from build123d import *

# Parameters (mm, degrees)
SKETCH1_W                    = 72.898
SKETCH1_H                    = 19.05
SKETCH1_R                    = 4.191
BOSS_EXTRUDE1_DEPTH          = 1.27
SKETCH7_W                    = 72.898
SKETCH7_H                    = 1.27
BOSS_EXTRUDE4_DEPTH          = 30.48
CUT_EXTRUDE2_DEPTH           = 50.267816331
SKETCH10_W                   = 1.27
SKETCH10_H                   = 27.94
BOSS_EXTRUDE5_DEPTH          = 8.89
SKETCH11_W                   = 1.27
SKETCH11_H                   = 27.94
BOSS_EXTRUDE6_DEPTH          = 11.43
SKETCH12_R                   = 2.5
CUT_EXTRUDE3_DEPTH           = 72.631264997
CUT_EXTRUDE5_DEPTH           = 72.631264997
CUT_EXTRUDE5_DEPTH_BACK      = 72.631264997
SKETCH14_W                   = 12.7
SKETCH14_H                   = 5.24
SKETCH15_W                   = 36.322
SKETCH15_H                   = 1.27
BOSS_EXTRUDE8_DEPTH          = 3.81
BOSS_EXTRUDE9_START          = 29.05
BOSS_EXTRUDE9_DEPTH          = 1.27
SKETCH17_R                   = 4.191
CUT_EXTRUDE6_DEPTH           = 1.27
CUT_EXTRUDE6_DRAFT           = -60
CUT_EXTRUDE6_PROFILE_2_DEPTH = 1.27
CUT_EXTRUDE6_PROFILE_2_DRAFT = -60


with BuildPart() as part:
    # Sketch1 → Boss-Extrude1 (new body)
    # profile 1 of 3: a face of its own
    with BuildSketch(Plane(origin=(0, 0, 0), x_dir=(1, 0, 0), z_dir=(0, 1, 0))):
        Rectangle(SKETCH1_W, SKETCH1_H)
        with Locations((28.829, 1.905)):
            Circle(SKETCH1_R, mode=Mode.SUBTRACT)
        with Locations((-28.829, 1.905)):
            Circle(SKETCH1_R, mode=Mode.SUBTRACT)
    # profile 2 of 3: a face of its own
    with BuildSketch(Plane(origin=(0, 0, 0), x_dir=(1, 0, 0), z_dir=(0, 1, 0))):
        with Locations((28.829, 1.905)):
            Circle(SKETCH1_R)
    # profile 3 of 3: a face of its own
    with BuildSketch(Plane(origin=(0, 0, 0), x_dir=(1, 0, 0), z_dir=(0, 1, 0))):
        with Locations((-28.829, 1.905)):
            Circle(SKETCH1_R)
    extrude(amount=BOSS_EXTRUDE1_DEPTH)

    # Cut-Extrude1 cone 1 section (through the dimple's axis) → Cut-Extrude1 (revolve, cut)
    with BuildSketch(Plane(origin=(-28.829, 0, -1.905), x_dir=(0, 0, -1), z_dir=(1, 0, 0))):
        Polygon((0, 0), (4.191, 0), (0, 2.419674978), align=None)
    revolve(axis=Axis((-28.829, 0, -1.905), (0, 1, 0)), mode=Mode.SUBTRACT)

    # Cut-Extrude1 cone 2 section (through the dimple's axis) → Cut-Extrude1 cone 2 (revolve, cut)
    with BuildSketch(Plane(origin=(28.829, 0, -1.905), x_dir=(0, 0, -1), z_dir=(1, 0, 0))):
        Polygon((0, 0), (4.191, 0), (0, 2.419674978), align=None)
    revolve(axis=Axis((28.829, 0, -1.905), (0, 1, 0)), mode=Mode.SUBTRACT)

    # Sketch7 → Boss-Extrude4 (add)
    with BuildSketch(Plane(origin=(0, 1.27, 0), x_dir=(1, 0, 0), z_dir=(0, 1, 0))):
        with Locations((0, -8.89)):
            Rectangle(SKETCH7_W, SKETCH7_H)
    extrude(amount=BOSS_EXTRUDE4_DEPTH)

    # Sketch8 → Cut-Extrude2 (cut, symmetric)
    with BuildSketch(Plane.XZ):
        Polygon((-36.449, 9.525), (-36.449, 3.354745169), (-18.161, 8.255), (-18.161, 9.525), align=None)
    cut_extrude2 = extrude(amount=CUT_EXTRUDE2_DEPTH, both=True, mode=Mode.SUBTRACT)

    # Mirror2: Cut-Extrude2 across plane
    add(cut_extrude2.mirror(Plane.ZY), mode=Mode.SUBTRACT)

    # Sketch10 → Boss-Extrude5 (add)
    with BuildSketch(Plane.ZY.offset(18.161)):
        with Locations((8.89, 17.78)):
            Rectangle(SKETCH10_W, SKETCH10_H)
    extrude(amount=BOSS_EXTRUDE5_DEPTH)

    # Sketch11 → Boss-Extrude6 (add)
    with BuildSketch(Plane(origin=(0, 0, 8.255), x_dir=(-1, 0, 0), z_dir=(0, 0, -1))):
        with Locations((26.416, 17.78)):
            Rectangle(SKETCH11_W, SKETCH11_H)
    extrude(amount=BOSS_EXTRUDE6_DEPTH)

    # Sketch12 → Cut-Extrude3 (cut, through all)
    with BuildSketch(Plane.ZY.offset(27.051)):
        with Locations((2.77876, 10.16)):
            Circle(SKETCH12_R)
        with Locations((2.77876, 20.16)):
            Circle(SKETCH12_R)
    extrude(amount=-CUT_EXTRUDE3_DEPTH, mode=Mode.SUBTRACT)

    # Sketch14 → Cut-Extrude5 (cut, two sides: drawn at the far end of the back side and taken through both)
    with BuildSketch(Plane.ZY.offset(27.051).offset(-CUT_EXTRUDE5_DEPTH_BACK)):
        with Locations((3.175, 29.13)):
            Rectangle(SKETCH14_W, SKETCH14_H)
    extrude(amount=CUT_EXTRUDE5_DEPTH + CUT_EXTRUDE5_DEPTH_BACK, mode=Mode.SUBTRACT)

    # Sketch15 → Boss-Extrude8 (add)
    with BuildSketch(Plane(origin=(0, 26.51, 0), x_dir=(1, 0, 0), z_dir=(0, 1, 0))):
        with Locations((0, -8.89)):
            Rectangle(SKETCH15_W, SKETCH15_H)
    extrude(amount=BOSS_EXTRUDE8_DEPTH)

    # Sketch16 → Boss-Extrude9 (add)
    with BuildSketch(Plane(origin=(0, 1.27, 0), x_dir=(1, 0, 0), z_dir=(0, 1, 0)).offset(BOSS_EXTRUDE9_START)):
        Polygon((-36.449, 9.525), (-36.449, -3.354745169), (-18.161, -8.255), (-18.161, -9.525), (18.161, -9.525), (18.161, -8.255), (36.449, -3.354745169), (36.449, 9.525), align=None)
    extrude(amount=-BOSS_EXTRUDE9_DEPTH)


with BuildPart() as cut_extrude6_tool:
    # Sketch17 → Cut-Extrude6 (with draft: the straight prism first)
    with BuildSketch(Plane(origin=(0, 30.32, 0), x_dir=(1, 0, 0), z_dir=(0, 1, 0))):
        with Locations((-28.829, 1.905)):
            Circle(SKETCH17_R)
    extrude(amount=-CUT_EXTRUDE6_DEPTH)
    # Cut-Extrude6: the draft: its side faces are tilted about the plane it starts from
    cut_extrude6_sides = [cut_extrude6_tool.faces().sort_by_distance(p)[0] for p in [
        (-33.02, 29.685, -1.905),
    ]]
    draft(cut_extrude6_sides, Plane(origin=(0, 30.32, 0), x_dir=(1, 0, 0), z_dir=(0, 1, 0)), CUT_EXTRUDE6_DRAFT)


with BuildPart() as part_1:
    add(part.part)

    # Cut-Extrude6: cut by cut_extrude6_tool
    add(cut_extrude6_tool.part, mode=Mode.SUBTRACT)


with BuildPart() as cut_extrude6_profile_2_tool:
    # Sketch17 → Cut-Extrude6 profile 2 (with draft: the straight prism first)
    with BuildSketch(Plane(origin=(0, 30.32, 0), x_dir=(1, 0, 0), z_dir=(0, 1, 0))):
        with Locations((28.829, 1.905)):
            Circle(SKETCH17_R)
    extrude(amount=-CUT_EXTRUDE6_PROFILE_2_DEPTH)
    # Cut-Extrude6 profile 2: the draft: its side faces are tilted about the plane it starts from
    cut_extrude6_profile_2_sides = [cut_extrude6_profile_2_tool.faces().sort_by_distance(p)[0] for p in [
        (24.638, 29.685, -1.905),
    ]]
    draft(cut_extrude6_profile_2_sides, Plane(origin=(0, 30.32, 0), x_dir=(1, 0, 0), z_dir=(0, 1, 0)), CUT_EXTRUDE6_PROFILE_2_DRAFT)


with BuildPart() as part_2:
    add(part_1.part)

    # Cut-Extrude6 profile 2: cut by cut_extrude6_profile_2_tool
    add(cut_extrude6_profile_2_tool.part, mode=Mode.SUBTRACT)


solid = part_2.part
Verification items for the finished model (mm, model axes). A direction names the side the tool comes from. Give positions to 0.01 mm unless a question says otherwise; leave off trailing zeros. Loops run counter-clockwise (first coordinate to the right, second up) from the corner with the lowest first, then second, coordinate; pieces in that order, holes last. Notation, with made-up numbers: (-11, -38.75) - (16, -38.75) arc R6 ccw to (16, -33.75) - close; hole circle Ø5 at (83.5, -30.75). An arc over 180 degrees is marked (long way). Write item = value, one per line. Start each with the question number.
Q1. Cross-section at D-D, the plane y = 17. Enter the section's corners in (x, z) (3 decimals).
Q2. Cross-section at C-C, the plane x = -14. Enter the section's corners in (y, z) (3 decimals), and give its area (3 significant figures).
Q3. Mould release check, pull along Y, two halves, no side actions. Record for faces 6 (the face through (-26.425, 8.639, 0.795)), 7 (the face through (-1, 0, 0)), 8 (the face through (-36.449, 30, -3)): released by +Y, released by -Y, zero draft, split by the parting line, or undercut.
Q4. Cross-section at A-A, the plane z = -7.25. Enter the section's corners in (x, y), and give its area (3 significant figures).
Q5. Thickness scan on line 1 (Y direction, x = -20, z = -7); line 2 (Y direction, x = -26.5, z = 5.75); line 3 (X direction, y = 11.5, z = 6.75). Record the ranges inside material, lowest first.
Q6. Depth check by flat-ended pin: P1, Ø1.5, axis at x = -10, z = 5.5, coming from the -Y side; P2, Ø2, axis at x = -29, y = 8, coming from the -Z side; P3, Ø1.4, axis at y = 2.5, z = 9, coming from the -X side; P4, Ø5, axis at x = 20.5, y = 23, coming from the -Z side (3 decimals). Enter the tip coordinate at first touch or a pass-through.
Q7. Cross-section at B-B, the plane y = 10.16. Enter the section's corners in (x, z) (3 decimals).
Q8. Tool access check on faces 1 (the face through (-18.161, 28, 9)), 2 (the face through (-26.42, 22.64, 2.45)), 3 (the face through (-25.781, 15, 3)), 4 (the face through (-1, 1.27, -1)), 5 (the face through (-26, 26.51, 5)). Record the directions out of +Z, -Z, +X, -X, +Y, -Y that give a thin tool (end or side, any length) a straight path to the whole face; none if there is none.
Answer key:
q1.outline = (-27.051, -3.175) - (-25.781, -3.175) - (-25.781, 8.255) - (18.161, 8.255) - (18.161, 9.525) - (-27.051, 9.525) - close
q2.outline = (0, -9.525) - (1.27, -9.525) - (1.27, 8.255) - (29.05, 8.255) - (29.05, -9.525) - (30.32, -9.525) - (30.32, 9.525) - (0, 9.525) - close
q2.area = 83.7 mm^2
q3.face_6 = undercut
q3.face_7 = released by -Y
q3.face_8 = zero draft
q4.outline = (-36.45, 0) - (36.45, 0) - (36.45, 1.27) - (-36.45, 1.27) - close; (-36.45, 29.05) - (36.45, 29.05) - (36.45, 30.32) - (-36.45, 30.32) - close
q4.area = 185 mm^2
q5.line_1 = 0 to 1.27, 29.05 to 30.32
q5.line_2 = 0 to 1.27, 3.81 to 26.51, 29.05 to 30.32
q5.line_3 = -27.05 to -25.78
q6.P1 = 0
q6.P2 = through
q6.P3 = -18.16
q6.P4 = 8.255
q7.outline = (-27.051, -3.175) - (-25.781, -3.175) - (-25.781, 0.279) - (-27.051, 0.279) - close; (-27.051, 5.279) - (-25.781, 5.279) - (-25.781, 8.255) - (18.161, 8.255) - (18.161, 9.525) - (-27.051, 9.525) - close
q8.face_1 = +Z, -X, +Y
q8.face_2 = +X, -X
q8.face_3 = -Z, +X
q8.face_4 = -Z, +X, -X
q8.face_5 = +Z, -Z, -X
